```python
from build123d import *

# Parameters (mm, degrees)
RESSALTO_EXTRUS_O1_DEPTH = 28
ESBO_O3_R                = 9
RESSALTO_EXTRUS_O2_DEPTH = 22
CHANFRO2_SIZE            = 0.5


with BuildPart() as part:
    # Esboço2 → Ressalto-extrusão1 (new body)
    with BuildSketch(Plane.XY):
        with BuildLine():
            Line((-3.024645143, -8.476527695), (-3.024645143, -4.976527695))
            Line((-3.024645143, -4.976527695), (2.975354857, -4.976527695))
            Line((2.975354857, -4.976527695), (2.975354857, -8.493954525))
            ThreePointArc((2.975354857, -8.493954525), (0.026140135, 8.999962038), (-3.024645143, -8.476527695))
        make_face()
    extrude(amount=RESSALTO_EXTRUS_O1_DEPTH)

    # Esboço3 → Ressalto-extrusão2 (add)
    with BuildSketch(Plane.XY.offset(28)):
        with Locations(Location((0, 0, 0), (0, 0, 250.362280418))):
            Circle(ESBO_O3_R)
    extrude(amount=RESSALTO_EXTRUS_O2_DEPTH)

    # Chanfro2
    chanfro2_edges = [part.edges().sort_by_distance(p)[0] for p in [
        (0.026140135, 8.999962038, 0),
    ]]
    chamfer(chanfro2_edges, length=CHANFRO2_SIZE)


solid = part.part
```
The model under review builds one solid part; all positions refer to its coordinate system, in mm. A direction names the side the tool comes from. Round coordinates to 2 decimals unless told otherwise and drop trailing zeros. Order: outer loops, then holes, each group sorted by start corner. A loop starts at its lowest first (then second) coordinate and runs counter-clockwise, first axis right, second up.
Item 1: Draft analysis for pull direction X (two halves, no side actions). For faces 1 (the flat face through (0, -4.977, 14)), 2 (the flat face through (0, 0, 0)), 3 (the conical face through (0.36, 8.63, 0.14)), state which applies: released by +X, released by -X, zero draft, split by the parting line, or undercut.
Working result:
face 1: undercut
face 2: zero draft
face 3: split by the parting line
Item 2: To check wall thickness, follow probe 1 along Y at (x, z) = (0.25, 24); probe 2 along Z at (x, y) = (-1, -7.75); probe 3 along Y at (x, z) = (0.25, 36.5). State the ranges of each line that lie inside material, in increasing order.
Working result:
probe 1: y = -4.98 to 9
probe 2: z = 28 to 50
probe 3: y = -9 to 9
Item 3: For pin 1 (1.1 mm diameter, centred on y = -7.5, z = 12, fed in from -X); pin 2 (4 mm diameter, centred on y = -7.5, z = 19.5, fed in from +X); pin 3 (5 mm diameter, centred on x = 1, z = 16, fed in from -Y), all flat-tipped, find the tip position at first contact; note any pin that passes through.
Working result:
pin 1: stops at x = -5.72
pin 2: stops at x = 7.12
pin 3: stops at y = -8.49
Item 4: Add section A-A, the plane x = 0. State the section outline as (y, z) points, and give its area (3 significant figures).
Working result:
outline: (-9, 28) - (-4.98, 28) - (-4.98, 0) - (8.5, 0) - (9, 0.5) - (9, 50) - (-9, 50) - close
area: 787 mm2
Item 5: Add section C-C, the plane z = 19. State the section outline as (x, y) points, and give its area (3 significant figures).
Working result:
outline: (-3.02, -8.48) - (-3.02, -4.98) - (2.98, -4.98) - (2.98, -8.49) arc R9 ccw (long way) to start
area: 231 mm2
Item 6: Machinability: for faces 4 (the flat face through (0, 0, 50)), 5 (the flat face through (2.975, -7, 14)), which of the approach directions +Z, -Z, +X, -X, +Y, -Y give a long, thin tool a straight path to every point of the face, cutting with its end or side? Answer none if there is none.
Working result:
face 4: +Z, +X, -X, +Y, -Y
face 5: -Z, -Y
Item 7: Add section B-B, the plane z = 39. State the section outline as (x, y) points, and give its area (3 significant figures).
Working result:
outline: circle Ø18 at (0, 0)
area: 254 mm2
